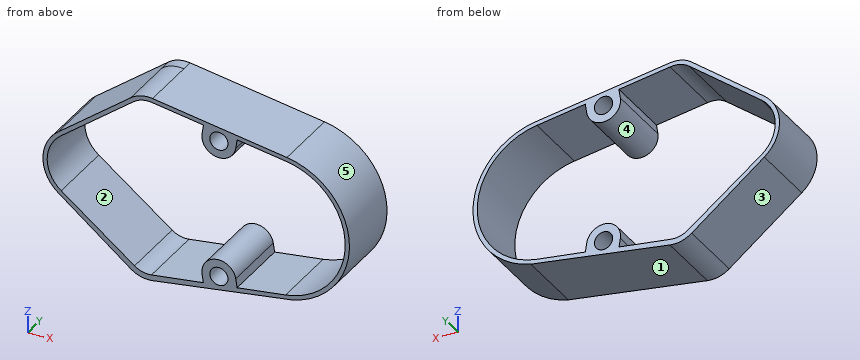
```python
from build123d import *
from build123d.topology import SkipClean

# Parameters (mm, degrees)
SKETCH1_R               = 1.6
SKETCH1_R_2             = 1
SKETCH1_R_3             = 5.5
SKETCH1_R_4             = 4.5
BOSS_EXTRUDE2_DEPTH     = 2
BOSS_EXTRUDE3_START     = -2
SKETCH2_R               = 1
BOSS_EXTRUDE3_DEPTH     = 2
SKETCH3_R               = 1
CUT_EXTRUDE1_DEPTH      = 103
BOSS_EXTRUDE4_OUTLINE_R = 1
BOSS_EXTRUDE4_DEPTH     = 10
SKETCH5_R               = 87.063932705
CUT_EXTRUDE2_DEPTH      = 2
SKETCH6_R               = 1
BOSS_EXTRUDE5_DEPTH     = 2
SKETCH7_R               = 1.6
BOSS_EXTRUDE6_DEPTH     = 12
SKETCH8_R               = 1.6
CUT_EXTRUDE3_DEPTH      = 12


# Read off the part's stored shape, not the designer's step: Boss-Extrude4
with BuildPart() as part:
    # Sketch1 → Boss-Extrude2 (new body)
    with BuildSketch(Plane(origin=(0, 0, 0), x_dir=(1, 0, 0), z_dir=(0, 1, 0))):
        with BuildLine():
            Line((12.313589515, -16.493996637), (35.979225245, -12.848450001))
            ThreePointArc((35.979225245, -12.848450001), (46.993067566, -0.424494085), (36.813648041, 12.691862933))
            Line((36.813648041, 12.691862933), (35.165189196, 12.947676785))
            Line((35.165189196, 12.947676785), (12.319067304, 16.493021261))
            ThreePointArc((12.319067304, 16.493021261), (11.720527595, 16.549330191), (11.119556233, 16.533395936))
            Line((11.119556233, 16.533395936), (-11.812019178, 14.541098507))
            ThreePointArc((-11.812019178, 14.541098507), (-13.247239988, 14.027709898), (-14.244912332, 12.87528787))
            Line((-14.244912332, 12.87528787), (-19.487592157, 2.204884721))
            ThreePointArc((-19.487592157, 2.204884721), (-19.693653105, -1.723258696), (-16.994761113, -4.584858569))
            Line((-16.994761113, -4.584858569), (9.557587922, -16.137143667))
            ThreePointArc((9.557587922, -16.137143667), (10.910298182, -16.51089082), (12.313589515, -16.493996637))
        make_face()
        with Locations(Location((11.552349036, -11.552285098, 0), (0, 0, 270))):
            Circle(SKETCH1_R, mode=Mode.SUBTRACT)
        with Locations(Location((25, -11, 0), (0, 0, 270))):
            Circle(SKETCH1_R_2, mode=Mode.SUBTRACT)
        with Locations(Location((-15, 0, 0), (0, 0, 270))):
            Circle(SKETCH1_R, mode=Mode.SUBTRACT)
        with Locations(Location((0, 0, 0), (0, 0, 270))):
            Circle(SKETCH1_R_3, mode=Mode.SUBTRACT)
        with Locations(Location((-11.552357038, 11.552357038, 0), (0, 0, 270))):
            Circle(SKETCH1_R, mode=Mode.SUBTRACT)
        with Locations(Location((11.552326466, 11.552160153, 0), (0, 0, 270))):
            Circle(SKETCH1_R, mode=Mode.SUBTRACT)
        with Locations(Location((14, 0, 0), (0, 0, 270))):
            Circle(SKETCH1_R_4, mode=Mode.SUBTRACT)
        with Locations(Location((34, 0, 0), (0, 0, 270))):
            Circle(SKETCH1_R_4, mode=Mode.SUBTRACT)
        with Locations(Location((25, 11, 0), (0, 0, 270))):
            Circle(SKETCH1_R_2, mode=Mode.SUBTRACT)
    extrude(amount=BOSS_EXTRUDE2_DEPTH)

    # Sketch2 → Boss-Extrude3 (add)
    with BuildSketch(Plane(origin=(0, 2, 0), x_dir=(1, 0, 0), z_dir=(0, 1, 0)).offset(BOSS_EXTRUDE3_START)):
        with Locations((25, 11)):
            Circle(SKETCH2_R)
        with Locations((25, -11)):
            Circle(SKETCH2_R)
    extrude(amount=BOSS_EXTRUDE3_DEPTH)

    # Sketch3 → Cut-Extrude1 (cut)
    with BuildSketch(Plane(origin=(0, 2, 0), x_dir=(1, 0, 0), z_dir=(0, 1, 0))):
        with Locations(Location((24, 13, 0), (0, 0, 270))):
            Circle(SKETCH3_R)
        with Locations(Location((24, -13, 0), (0, 0, 270))):
            Circle(SKETCH3_R)
    extrude(amount=-CUT_EXTRUDE1_DEPTH, mode=Mode.SUBTRACT)

    # Boss-Extrude4 outline → Boss-Extrude4 (add)
    with SkipClean():  # the faces are left unmerged after this step: merging them gives an invalid solid
        with BuildSketch(Plane(origin=(0, 2, 0), x_dir=(1, 0, 0), z_dir=(0, 1, 0))):
            with BuildLine():
                ThreePointArc((8.453372169, -15.47610242), (10.277484332, -16.387026041), (12.313589515, -16.493996637))
                Line((12.313589515, -16.493996637), (35.979225245, -12.848450001))
                ThreePointArc((35.979225245, -12.848450001), (46.993067566, -0.424494085), (36.813648041, 12.691862933))
                Line((36.813648041, 12.691862933), (12.319067304, 16.493021261))
                ThreePointArc((12.319067304, 16.493021261), (10.294223964, 16.391290043), (8.476229775, 15.493940099))
                Line((8.476229775, 15.493940099), (-4.306535369, 5.518491924))
                ThreePointArc((-4.306535369, 5.518491924), (-7, 0), (-4.306535369, -5.518491924))
                Line((-4.306535369, -5.518491924), (8.453372169, -15.47610242))
            make_face()
            with Locations((24, -13)):
                Circle(BOSS_EXTRUDE4_OUTLINE_R, mode=Mode.SUBTRACT)
            with BuildLine():
                Line((35.738243971, -12.126046672), (26.117255626, -13.608064851))
                Line((26.117255626, -13.608064851), (25.976685738, -12.695511096))
                ThreePointArc((25.976685738, -12.695511096), (23.695511096, -11.023314262), (22.023314262, -13.304488904))
                Line((22.023314262, -13.304488904), (22.16388415, -14.217042659))
                Line((22.16388415, -14.217042659), (12.27862862, -15.739768587))
                ThreePointArc((12.27862862, -15.739768587), (10.519552717, -15.67488522), (8.937649363, -14.902784407))
                Line((8.937649363, -14.902784407), (-3.845146577, -4.927204867))
                ThreePointArc((-3.845146577, -4.927204867), (-6.249813783, 0.048245957), (-3.768620923, 4.985979978))
                Line((-3.768620923, 4.985979978), (9.140409076, 14.743187339))
                ThreePointArc((9.140409076, 14.743187339), (10.553310252, 15.425397379), (12.119916334, 15.511685597))
                Line((12.119916334, 15.511685597), (22.133828609, 14.076211769))
                Line((22.133828609, 14.076211769), (22.020237278, 13.283794934))
                ThreePointArc((22.020237278, 13.283794934), (23.716205066, 11.020237278), (25.979762722, 12.716205066))
                Line((25.979762722, 12.716205066), (26.093354053, 13.508621901))
                Line((26.093354053, 13.508621901), (35.738243971, 12.126046672))
                ThreePointArc((35.738243971, 12.126046672), (46.25, 0), (35.738243971, -12.126046672))
            make_face(mode=Mode.SUBTRACT)
            with Locations((24, 13)):
                Circle(BOSS_EXTRUDE4_OUTLINE_R, mode=Mode.SUBTRACT)
        extrude(amount=BOSS_EXTRUDE4_DEPTH)
    add(part.part.scale(1), mode=Mode.REPLACE)  # the faces are merged on a copy

    # Sketch5 → Cut-Extrude2 (cut)
    with BuildSketch(Plane(origin=(0, 0, 0), x_dir=(-1, 0, 0), z_dir=(0, -1, 0))):
        Circle(SKETCH5_R)
    extrude(amount=-CUT_EXTRUDE2_DEPTH, mode=Mode.SUBTRACT)

    # Sketch6 → Boss-Extrude5 (add)
    with SkipClean():  # the faces are left unmerged after this step: merging them gives an invalid solid
        with BuildSketch(Plane(origin=(0, 12, 0), x_dir=(1, 0, 0), z_dir=(0, 1, 0))):
            with BuildLine():
                Line((-4.306535369, 5.518491924), (8.476229775, 15.493940099))
                ThreePointArc((8.476229775, 15.493940099), (10.294223964, 16.391290043), (12.319067304, 16.493021261))
                Line((12.319067304, 16.493021261), (36.813648041, 12.691862933))
                ThreePointArc((36.813648041, 12.691862933), (46.993067566, -0.424494085), (35.979225245, -12.848450001))
                Line((35.979225245, -12.848450001), (12.313589515, -16.493996637))
                ThreePointArc((12.313589515, -16.493996637), (10.277484331, -16.387026041), (8.453372169, -15.47610242))
                Line((8.453372169, -15.47610242), (-4.306535369, -5.518491924))
                ThreePointArc((-4.306535369, -5.518491924), (-7, 0), (-4.306535369, 5.518491924))
            make_face()
            with Locations(Location((24, -13, 0), (0, 0, 270))):
                Circle(SKETCH6_R, mode=Mode.SUBTRACT)
            with Locations(Location((24, 13, 0), (0, 0, 270))):
                Circle(SKETCH6_R, mode=Mode.SUBTRACT)
            with BuildLine():
                Line((35.738243971, 12.126046672), (26.093354053, 13.508621901))
                Line((26.093354053, 13.508621901), (25.979762722, 12.716205066))
                ThreePointArc((25.979762722, 12.716205066), (23.716205066, 11.020237278), (22.020237278, 13.283794934))
                Line((22.020237278, 13.283794934), (22.133828609, 14.076211769))
                Line((22.133828609, 14.076211769), (12.119916334, 15.511685597))
                ThreePointArc((12.119916334, 15.511685597), (10.553310252, 15.425397379), (9.140409076, 14.743187339))
                Line((9.140409076, 14.743187339), (-3.768620923, 4.985979978))
                ThreePointArc((-3.768620923, 4.985979978), (-6.249813783, 0.048245957), (-3.845146577, -4.927204867))
                Line((-3.845146577, -4.927204867), (8.937649363, -14.902784407))
                ThreePointArc((8.937649363, -14.902784407), (10.519552717, -15.67488522), (12.27862862, -15.739768587))
                Line((12.27862862, -15.739768587), (22.16388415, -14.217042659))
                Line((22.16388415, -14.217042659), (22, -13))
                ThreePointArc((22, -13), (23.847309916, -11.005837083), (25.976685738, -12.695511096))
                Line((25.976685738, -12.695511096), (26.117255626, -13.608064851))
                Line((26.117255626, -13.608064851), (35.738243971, -12.126046672))
                ThreePointArc((35.738243971, -12.126046672), (46.25, 0), (35.738243971, 12.126046672))
            make_face(mode=Mode.SUBTRACT)
        extrude(amount=BOSS_EXTRUDE5_DEPTH)

    # Sketch7 → Boss-Extrude6 (add)
    # profile 1 of 2: a face of its own
    with BuildSketch(Plane(origin=(0, 14, 0), x_dir=(1, 0, 0), z_dir=(0, 1, 0))):
        with BuildLine():
            Line((22.591660568, 14.898882792), (26.144897094, 14.347478595))
            Line((26.144897094, 14.347478595), (27.332795496, 14.163136191))
            Line((27.332795496, 14.163136191), (26.964516665, 11.789955497))
            ThreePointArc((26.964516665, 11.789955497), (23.539955497, 9.285483335), (21.035483335, 12.710044503))
            Line((21.035483335, 12.710044503), (21.403762166, 15.083225196))
            Line((21.403762166, 15.083225196), (22.591660568, 14.898882792))
        make_face()
        with Locations((24, 12.25)):
            Circle(SKETCH7_R, mode=Mode.SUBTRACT)
    # profile 2 of 2: a face of its own
    with BuildSketch(Plane(origin=(0, 14, 0), x_dir=(1, 0, 0), z_dir=(0, 1, 0))):
        with BuildLine():
            Line((26.126412864, -14.366215568), (21.402696028, -15.093875294))
            Line((21.402696028, -15.093875294), (21.034973077, -12.706744287))
            ThreePointArc((21.034973077, -12.706744287), (23.543255713, -9.284973077), (26.965026923, -11.793255713))
            Line((26.965026923, -11.793255713), (27.332749874, -14.18038672))
            Line((27.332749874, -14.18038672), (26.126412864, -14.366215568))
        make_face()
        with Locations((24, -12.25)):
            Circle(SKETCH7_R, mode=Mode.SUBTRACT)
    extrude(amount=-BOSS_EXTRUDE6_DEPTH)

    # Sketch8 → Cut-Extrude3 (cut)
    with BuildSketch(Plane(origin=(0, 14, 0), x_dir=(1, 0, 0), z_dir=(0, 1, 0))):
        with Locations(Location((24, -12.25, 0), (0, 0, 270))):
            Circle(SKETCH8_R)
        with Locations(Location((24, 12.25, 0), (0, 0, 270))):
            Circle(SKETCH8_R)
    extrude(amount=-CUT_EXTRUDE3_DEPTH, mode=Mode.SUBTRACT)


solid = part.part
```
The model under review builds one solid part; all positions refer to its coordinate system, in mm. Face numbers are marked on the shaded views. A direction names the side the tool comes from. Round coordinates to 2 decimals unless told otherwise and drop trailing zeros. Loops run counter-clockwise (first coordinate to the right, second up) from the corner with the lowest first, then second, coordinate; pieces in that order, holes last.
1) Consider section C-C on x = 24. State the section outline as (y, z) points, then the cut area to 3 significant figures.
Values follow:
outline: (2, -14.68) - (14, -14.68) - (14, -13.85) - (2, -13.85) - close; (2, -10.65) - (14, -10.65) - (14, -9.25) - (2, -9.25) - close; (2, 9.25) - (14, 9.25) - (14, 10.65) - (2, 10.65) - close; (2, 13.85) - (14, 13.85) - (14, 14.69) - (2, 14.69) - close
area: 53.7 mm2
2) Consider section D-D on y = 11.25. Give the number of separate pieces and of enclosed holes in the cut face, then the cut area to 3 significant figures.
Values follow:
separate pieces: 1
enclosed holes: 3
area: 139 mm2
3) Tool access review of the marked faces 1 and 2: name each direction out of +Z, -Z, +X, -X, +Y, -Y from which nothing blocks a thin tool from reaching the whole face with its end or side.
Values follow:
face 1: -Z, +X, +Y, -Y
face 2: +Y, -Y
4) Consider section A-A on z = 0. State the section outline as (x, y) points.
Values follow:
outline: (-7, 2) - (-6.25, 2) - (-6.25, 14) - (-7, 14) - close; (46.25, 2) - (47, 2) - (47, 14) - (46.25, 14) - close
5) Consider section B-B on x = -2. State the section outline as (y, z) points.
Values follow:
outline: (2, -7.32) - (14, -7.32) - (14, -6.32) - (2, -6.32) - close; (2, 6.37) - (14, 6.37) - (14, 7.32) - (2, 7.32) - close
6) Clearance check with flat-ended pins moving along their axes: P1, Ø1, axis at y = 3.5, z = 12, coming from the +X side; P2, Ø2, axis at x = 40.5, y = 6, coming from the +Z side; P3, Ø3, axis at y = 10.5, z = 10, coming from the -X side. State where each tip first meets the part, or that it passes through.
Values follow:
P1: stops at x = 40.06
P2: stops at z = 11.78
P3: stops at x = -0.49
7) The part is to be moulded in two halves that separate along X. For the marked faces 3, 4 and 5, say which applies: pulls with the +X half, pulls with the -X half, needs draft (parallel to the pull), parting line crosses it, or undercut.
Values follow:
face 3: pulls with the -X half
face 4: undercut
face 5: pulls with the +X half
8) Wall thickness on line 1 along Z through (x, y) = (24, 7); line 2 along X through (y, z) = (10.75, 6.5); line 3 along X through (y, z) = (3.5, -6): over which ranges is each line inside the solid? List them lowest first.
Values follow:
line 1: z = -14.68 to -13.85, -10.65 to -9.25, 9.25 to 10.65, 13.85 to 14.69
line 2: x = -3.05 to -1.83, 44.38 to 45.26
line 3: x = -3.69 to -2.43, 44.68 to 45.53
